from build123d import *

# Parameters (mm, degrees)
F1_DEPTH = 25.4
F2_R     = 6.35
F3_DEPTH = 25.4
F4_R     = 6.35
F5_DEPTH = 25.4
F6_R     = 6.35
F7_DEPTH = 25.4


with BuildPart() as f1:
    # F0 (on Front) → F1 (new body)
    with BuildSketch(Plane.XZ):
        Polygon((-31.75, 12.404651), (-31.75, -0.295349), (44.449428, -2e-06), (44.449428, 12.404651), (19.049428, 12.404651), (19.049428, 44.154651), (-6.350572, 44.154651), (-6.35, 12.404651), align=None)
    extrude(amount=F1_DEPTH)

    # F2 (on face) → F3 (cut)
    with BuildSketch(Plane.XY.offset(12.404651)):
        with Locations((-19.050572, -12.7)):
            Circle(F2_R)
        with BuildLine():
            ThreePointArc((-31.75, -12.579426), (-27.988098, -3.677215), (-19.050572, 0))
            Line((-19.050572, 0), (-31.75, 0))
            Line((-31.75, 0), (-31.75, -12.579426))
        make_face()
        with BuildLine():
            ThreePointArc((-19.050572, -25.4), (-27.988098, -21.722785), (-31.75, -12.820574))
            Line((-31.75, -12.820574), (-31.75, -25.4))
            Line((-31.75, -25.4), (-19.050572, -25.4))
        make_face()
    extrude(amount=-F3_DEPTH, mode=Mode.SUBTRACT)

    # F4 (on face) → F5 (cut)
    with BuildSketch(Plane.XY.offset(12.404651)):
        with Locations((31.749428, -12.7)):
            Circle(F4_R)
        with BuildLine():
            ThreePointArc((31.749428, 0), (40.729684, -3.719744), (44.449428, -12.7))
            Line((44.449428, -12.7), (44.449428, 0))
            Line((44.449428, 0), (31.749428, 0))
        make_face()
        with BuildLine():
            ThreePointArc((44.449428, -12.7), (40.729684, -21.680256), (31.749428, -25.4))
            Line((31.749428, -25.4), (44.449428, -25.4))
            Line((44.449428, -25.4), (44.449428, -12.7))
        make_face()
    extrude(amount=-F5_DEPTH, mode=Mode.SUBTRACT)

    # F6 (on face) → F7 (cut)
    with BuildSketch(Plane.YZ.offset(19.049428)):
        with Locations((-12.295053, 31.461109)):
            Circle(F6_R)
        with BuildLine():
            ThreePointArc((-12.7, 44.154651), (-3.719744, 40.434907), (0, 31.454651))
            Line((0, 31.454651), (0, 44.154651))
            Line((0, 44.154651), (-12.7, 44.154651))
        make_face()
        with BuildLine():
            ThreePointArc((-25.4, 31.454651), (-21.680256, 40.434907), (-12.7, 44.154651))
            Line((-12.7, 44.154651), (-25.4, 44.154651))
            Line((-25.4, 44.154651), (-25.4, 31.454651))
        make_face()
    extrude(amount=-F7_DEPTH, mode=Mode.SUBTRACT)


solid = f1.part
Can you work these out from the model? Positions are in its coordinate system, mm. A direction names the side the tool comes from. Round coordinates to 2 decimals unless told otherwise and drop trailing zeros. Loops run counter-clockwise (first coordinate to the right, second up) from the corner with the lowest first, then second, coordinate; pieces in that order, holes last. Notation, with made-up numbers: (32.5, 82) - (79.5, 82) arc R22 cw to (79.5, 118) - close; hole circle Ø8 at (75, 86.25). An arc over 180 degrees is marked (long way). Write item = value, one per line. Start each with the question number.
(1) For P1, Ø3, axis at x = 12.5, y = -16.5, coming from the -Z side; P2, Ø2, axis at x = -11, y = -4.5, coming from the -Z side; P3, Ø1.5, axis at y = -3, z = 13.5, coming from the +X side, each with a flat end and sliding along its axis, tell me the tip position at first contact or that it passes through.
(2) If we section it at B-B (y = -11.25): Please give me the cut outline in (x, z), and give its area (3 significant figures).
(3) If I drill on probe 1 along X at (y, z) = (-12.7, 4.75); probe 2 along Y at (x, z) = (-19.5, 4); probe 3 along X at (y, z) = (-13.25, 5.5), over which ranges is the centre line in solid material (lowest first)? Write a range as [from, to].
(4) For faces 4 (the face through (-28.09, -3.78, 6.14)), 5 (the face through (23, -13, 12.405)), 6 (the face through (-13, -10, 12.405)), which set-ups out of +Z, -Z, +X, -X, +Y, -Y let a thin tool reach every point of the face, with its end or its side?
(5) If we section it at A-A (z = 34.5): Please give me the cut outline in (x, y), and give its area (3 significant figures).
(6) If we section it at D-D (x = 0): Please give me the cut outline in (y, z).
(7) If we mould it in two halves opening along Y, with no side actions, what happens to faces 1 (the face through (-27.89, -21.82, 6.14)), 2 (the face through (6, 0, 12)), 3 (the face through (-20.43, -18.9, 6.16))? For each: released by +Y, released by -Y, zero draft, split by the parting line, or undercut.
(8) If we section it at C-C (x = -16.5): Please give me the cut outline in (y, z), and give its area (3 significant figures).
Ans:
q1.P1 = -0.13
q1.P2 = -0.22
q1.P3 = 19.05
q2.outline = (-31.67, -0.3) - (-25.23, -0.27) - (-25.23, 12.4) - (-31.67, 12.4) - close; (-12.87, -0.22) - (25.57, -0.07) - (25.57, 12.4) - (19.05, 12.4) - (19.05, 25.2) - (-6.35, 25.2) - (-6.35, 12.4) - (-12.87, 12.4) - close; (-6.35, 37.72) - (19.05, 37.72) - (19.05, 44.07) - (-6.35, 44.07) - close; (37.93, -0.03) - (44.37, 0) - (44.37, 12.4) - (37.93, 12.4) - close
q2.area = 1,130 mm²
q3.probe_1 = [-31.75, -25.4], [-12.7, 25.4], [38.1, 44.45]
q3.probe_2 = [-25.39, -19.03], [-6.37, -0.01]
q3.probe_3 = [-31.74, -25.38], [-12.72, 25.42], [38.08, 44.44]
q4.face_4 = +Z, -Z, -X, +Y
q4.face_5 = +Z, +X, +Y, -Y
q4.face_6 = +Z, -X, +Y, -Y
q5.outline = (-6.35, -25.03) - (19.05, -25.03) - (19.05, -17.87) - (-6.35, -17.87) - close; (-6.35, -6.72) - (19.05, -6.72) - (19.05, -0.37) - (-6.35, -0.37) - close
q5.area = 343 mm²
q6.outline = (-25.4, -0.17) - (0, -0.17) - (0, 31.45) arc R12.7 ccw to (-25.4, 31.45) - close; hole circle Ø12.7 at (-12.3, 31.46)
q7.face_1 = released by -Y
q7.face_2 = released by +Y
q7.face_3 = undercut
q8.outline = (-25.4, -0.24) - (-18.52, -0.24) - (-18.52, 12.4) - (-25.4, 12.4) - close; (-6.88, -0.24) - (0, -0.24) - (0, 12.4) - (-6.88, 12.4) - close
q8.area = 174 mm²
